For this review, take the finished solid that the model builds, in its own axes (mm). Face numbers are marked on the shaded views. A direction names the side the tool comes from. Give positions to 0.01 mm unless a question says otherwise; leave off trailing zeros. Order: outer loops, then holes, each group sorted by start corner. A loop starts at its lowest first (then second) coordinate and runs counter-clockwise, first axis right, second up. Notation, with made-up numbers: (48, 62.5) - (66, 62.5) arc R15 cw to (66, 73.5) - close; hole circle Ø1 at (50.25, 22). An arc over 180 degrees is marked (long way). One line per item, written item: value.
```python
from build123d import *

# Parameters (mm, degrees)
SKETCH1_R           = 12.7
BOSS_EXTRUDE1_DEPTH = 31.75
SKETCH2_R           = 3.175
CUT_EXTRUDE1_DEPTH  = 15.875
SKETCH3_R           = 12.7
SKETCH3_R_2         = 6.35
CUT_EXTRUDE2_DEPTH  = 44.45
SKETCH8_W           = 1.35255
SKETCH8_H           = 12.7
SKETCH4_R           = 1.8288
CUT_EXTRUDE3_DEPTH  = 48.941448757
SKETCH10_R          = 2.921
CUT_EXTRUDE5_DEPTH  = 9.525
CIRPATTERN1_COUNT   = 4


with BuildPart() as part:
    # Sketch1 → Boss-Extrude1 (new, symmetric)
    with BuildSketch(Plane(origin=(0, 0, 0), x_dir=(0, 0, -1), z_dir=(1, 0, 0))):
        Circle(SKETCH1_R)
    extrude(amount=BOSS_EXTRUDE1_DEPTH, both=True)

    # Sketch2 → Cut-Extrude1 (cut)
    with BuildSketch(Plane(origin=(31.75, 0, 0), x_dir=(0, 0, -1), z_dir=(1, 0, 0))):
        Circle(SKETCH2_R)
    extrude(amount=-CUT_EXTRUDE1_DEPTH, mode=Mode.SUBTRACT)

    # Sketch3 → Cut-Extrude2 (cut)
    with BuildSketch(Plane(origin=(31.75, 0, 0), x_dir=(0, 0, -1), z_dir=(1, 0, 0))):
        Circle(SKETCH3_R)
        Circle(SKETCH3_R_2, mode=Mode.SUBTRACT)
    extrude(amount=-CUT_EXTRUDE2_DEPTH, mode=Mode.SUBTRACT)

    # Sketch8 → #6-32 Tapped Hole2 (revolve, cut)
    with BuildSketch(Plane(origin=(25.4, 0, 0), x_dir=(0, 0, -1), z_dir=(1, 0, 0))):
        with Locations((0.676275, 6.35)):
            Rectangle(SKETCH8_W, SKETCH8_H)
    revolve(axis=Axis((25.4, -6.35, 0), (0, 1, 0)), mode=Mode.SUBTRACT)

    # Sketch4 → Cut-Extrude3 (cut, through all)
    with BuildSketch(Plane(origin=(-12.7, 0, 0), x_dir=(0, 0, -1), z_dir=(1, 0, 0))):
        with Locations((9.525, 0)):
            Circle(SKETCH4_R)
    cut_extrude3 = extrude(amount=-CUT_EXTRUDE3_DEPTH, mode=Mode.SUBTRACT)

    # Sketch10 → Cut-Extrude5 (cut)
    with BuildSketch(Plane.ZY.offset(31.75)):
        with Locations((-9.525, 0)):
            Circle(SKETCH10_R)
    cut_extrude5 = extrude(amount=-CUT_EXTRUDE5_DEPTH, mode=Mode.SUBTRACT)

    # CirPattern1: Cut-Extrude3, Cut-Extrude5 ×4 about axis
    cirpattern1_axis = Axis((0, 0, 0), (1, 0, 0))
    add([cut_extrude3.rotate(cirpattern1_axis, i * 360 / CIRPATTERN1_COUNT) for i in range(1, CIRPATTERN1_COUNT)], mode=Mode.SUBTRACT)
    add([cut_extrude5.rotate(cirpattern1_axis, i * 360 / CIRPATTERN1_COUNT) for i in range(1, CIRPATTERN1_COUNT)], mode=Mode.SUBTRACT)


solid = part.part
```
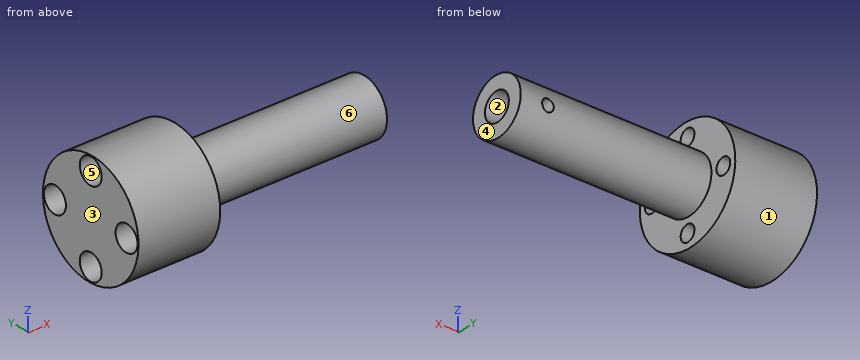
(1) Take a section at C-C (x = -27.5). Write out the cut boundary in (y, z) (3 decimals), then the cut area to 3 significant figures.
Answers below:
outline: circle Ø25.4 at (0, 0); hole circle Ø5.842 at (-9.525, 0); hole circle Ø5.842 at (0, -9.525); hole circle Ø5.842 at (0, 9.525); hole circle Ø5.842 at (9.525, 0)
area: 399 mm^2
(2) Take a section at D-D (y = 9.5). Write out the cut boundary in (x, z) (3 decimals).
Answers below:
outline: (-31.75, -8.429) - (-12.7, -8.429) - (-12.7, -1.829) - (-22.225, -1.829) - (-22.225, -2.921) - (-31.75, -2.921) - close; (-31.75, 2.921) - (-22.225, 2.921) - (-22.225, 1.829) - (-12.7, 1.829) - (-12.7, 8.429) - (-31.75, 8.429) - close
(3) For P1, Ø2, axis at x = 0.5, z = -6.5, coming from the +Y side; P2, Ø10, axis at x = 2.5, z = 8, coming from the +Y side; P3, Ø2, axis at y = 0, z = -9.525, coming from the -X side; P4, Ø6, axis at y = -9.525, z = 0, coming from the +X side, all flat-tipped, find the tip position at first contact; note any pin that passes through.
Answers below:
P1: stops at y = 3.17
P2: stops at y = 5.6
P3: passes through
P4: stops at x = -12.7
(4) Machinability: for the marked faces 4, 5 and 6, which of the approach directions +Z, -Z, +X, -X, +Y, -Y give a long, thin tool a straight path to every point of the face, cutting with its end or side? Answer none if there is none.
Answers below:
face 4: +Z, -Z, +X, +Y, -Y
face 5: -X
face 6: +X
(5) Draft analysis for pull direction Y (two halves, no side actions). For the marked faces 1, 2 and 3, state which applies: pulls with the +Y half, pulls with the -Y half, needs draft (parallel to the pull), parting line crosses it, or undercut.
Answers below:
face 1: parting line crosses it
face 2: undercut
face 3: needs draft
(6) Take a section at A-A (y = 0). Write out the cut boundary in (x, z) (3 decimals), then the cut area to 3 significant figures.
Answers below:
outline: (-31.75, -12.7) - (-12.7, -12.7) - (-12.7, -11.354) - (-22.225, -11.354) - (-22.225, -12.446) - (-31.75, -12.446) - close; (-31.75, -6.604) - (-22.225, -6.604) - (-22.225, -7.696) - (-12.7, -7.696) - (-12.7, -6.35) - (31.75, -6.35) - (31.75, -3.175) - (15.875, -3.175) - (15.875, 3.175) - (31.75, 3.175) - (31.75, 6.35) - (-12.7, 6.35) - (-12.7, 7.696) - (-22.225, 7.696) - (-22.225, 6.604) - (-31.75, 6.604) - close; (-31.75, 12.446) - (-22.225, 12.446) - (-22.225, 11.354) - (-12.7, 11.354) - (-12.7, 12.7) - (-31.75, 12.7) - close
area: 767 mm^2
(7) Wall thickness on line 1 (Z direction, x = -15.5, y = -0.75); line 2 (X direction, y = 6.5, z = -0.5); line 3 (Z direction, x = 22.5, y = -1.5): over which ranges is each line inside the solid? List them lowest first. Write a range as from..to.
Answers below:
line 1: z = -12.68..-11.19, -7.86..7.86, 11.19..12.68
line 2: x = -31.75..-12.7
line 3: z = -6.17..-2.8, 2.8..6.17
(8) Take a section at B-B (z = 0). Give the number of separate pieces and of enclosed holes in the cut face, then the cut area to 3 significant figures.
Answers below:
separate pieces: 4
enclosed holes: 0
area: 758 mm^2
